```python
from build123d import *

# Parameters (mm, degrees)
F0_W     = 78.4
F0_H     = 24.4
F0_R     = 1
F0_R_2   = 4.1
F1_DEPTH = 1.5
F2_W     = 25
F2_H     = 1.5
F3_DEPTH = 40
F4_R     = 1
F4_R_2   = 4.1
F5_DEPTH = 1.5
F6_R     = 5


with BuildPart() as f1:
    # F0 (on Top) → F1 (new body)
    with BuildSketch(Plane.XY):
        Rectangle(F0_W, F0_H)
        with Locations((-36.2, -7.2)):
            Circle(F0_R, mode=Mode.SUBTRACT)
        with Locations((-4.6, -7.2)):
            Circle(F0_R, mode=Mode.SUBTRACT)
        with Locations((4.6, -7.2)):
            Circle(F0_R, mode=Mode.SUBTRACT)
        with Locations((36.2, -7.2)):
            Circle(F0_R, mode=Mode.SUBTRACT)
        with Locations((-30, 0)):
            Circle(F0_R_2, mode=Mode.SUBTRACT)
        with BuildLine():
            ThreePointArc((-22.5, 4.8), (-21.035534, 8.335534), (-17.5, 9.8))
            Line((-17.5, 9.8), (-7.8, 9.8))
            ThreePointArc((-7.8, 9.8), (-7.092893, 9.507107), (-6.8, 8.8))
            Line((-6.8, 8.8), (-6.8, 5.59017))
            ThreePointArc((-6.8, 5.59017), (-6.712871, 5.181922), (-6.466667, 4.844814))
            ThreePointArc((-6.466667, 4.844814), (-4.3, 0), (-6.466667, -4.844814))
            ThreePointArc((-6.466667, -4.844814), (-6.712871, -5.181922), (-6.8, -5.59017))
            Line((-6.8, -5.59017), (-6.8, -8.8))
            ThreePointArc((-6.8, -8.8), (-7.092893, -9.507107), (-7.8, -9.8))
            Line((-7.8, -9.8), (-17.5, -9.8))
            ThreePointArc((-17.5, -9.8), (-21.035534, -8.335534), (-22.5, -4.8))
            Line((-22.5, -4.8), (-22.5, 4.8))
        make_face(mode=Mode.SUBTRACT)
        with Locations((-36.2, 7.2)):
            Circle(F0_R, mode=Mode.SUBTRACT)
        with Locations((-4.6, 7.2)):
            Circle(F0_R, mode=Mode.SUBTRACT)
        with BuildLine():
            Line((6.8, 5.59017), (6.8, 8.8))
            ThreePointArc((6.8, 8.8), (7.092893, 9.507107), (7.8, 9.8))
            Line((7.8, 9.8), (17.5, 9.8))
            ThreePointArc((17.5, 9.8), (21.035534, 8.335534), (22.5, 4.8))
            Line((22.5, 4.8), (22.5, -4.8))
            ThreePointArc((22.5, -4.8), (21.035534, -8.335534), (17.5, -9.8))
            Line((17.5, -9.8), (7.8, -9.8))
            ThreePointArc((7.8, -9.8), (7.092893, -9.507107), (6.8, -8.8))
            Line((6.8, -8.8), (6.8, -5.59017))
            ThreePointArc((6.8, -5.59017), (6.712871, -5.181922), (6.466667, -4.844814))
            ThreePointArc((6.466667, -4.844814), (4.3, 0), (6.466667, 4.844814))
            ThreePointArc((6.466667, 4.844814), (6.712871, 5.181922), (6.8, 5.59017))
        make_face(mode=Mode.SUBTRACT)
        with Locations((30, 0)):
            Circle(F0_R_2, mode=Mode.SUBTRACT)
        with Locations((4.6, 7.2)):
            Circle(F0_R, mode=Mode.SUBTRACT)
        with Locations((36.2, 7.2)):
            Circle(F0_R, mode=Mode.SUBTRACT)
    extrude(amount=F1_DEPTH)

    # F2 (on Top) → F3 (join)
    with BuildSketch(Plane.XY):
        with Locations((0, 12.95)):
            Rectangle(F2_W, F2_H)
    extrude(amount=F3_DEPTH)

    # F4 (on face) → F5 (cut, through all)
    with BuildSketch(Plane(origin=(0, 13.7, 0), x_dir=(-1, 0, 0), z_dir=(0, 1, 0))):
        with Locations((7.2, 37)):
            Circle(F4_R)
        with Locations((7.2, 5.4)):
            Circle(F4_R)
        with Locations((0, 11.6)):
            Circle(F4_R_2)
        with BuildLine():
            ThreePointArc((9.8, 33.9), (9.507107, 34.607107), (8.8, 34.9))
            Line((8.8, 34.9), (5.499091, 34.9))
            ThreePointArc((5.499091, 34.9), (5.099091, 34.983485), (4.765879, 35.22))
            ThreePointArc((4.765879, 35.22), (0, 37.3), (-4.765879, 35.22))
            ThreePointArc((-4.765879, 35.22), (-5.099091, 34.983485), (-5.499091, 34.9))
            Line((-5.499091, 34.9), (-8.8, 34.9))
            ThreePointArc((-8.8, 34.9), (-9.507107, 34.607107), (-9.8, 33.9))
            Line((-9.8, 33.9), (-9.8, 24.2))
            ThreePointArc((-9.8, 24.2), (-8.335534, 20.664466), (-4.8, 19.2))
            Line((-4.8, 19.2), (4.8, 19.2))
            ThreePointArc((4.8, 19.2), (8.335534, 20.664466), (9.8, 24.2))
            Line((9.8, 24.2), (9.8, 33.9))
        make_face()
        with Locations((-7.2, 37)):
            Circle(F4_R)
        with Locations((-7.2, 5.4)):
            Circle(F4_R)
    extrude(amount=-F5_DEPTH, mode=Mode.SUBTRACT)

    # F6
    f6_edges = [f1.edges().sort_by_distance(p)[0] for p in [
        (-39.2, 12.2, 0.75),
        (-39.2, -12.2, 0.75),
        (39.2, 12.2, 0.75),
        (39.2, -12.2, 0.75),
        (-12.5, 12.95, 40),
        (12.5, 12.95, 40),
    ]]
    fillet(f6_edges, radius=F6_R)


solid = f1.part
```
CAD build for the part. Positions are in the model's coordinates, mm. A direction names the side the tool comes from. Coordinates: 2 decimals unless noted, no trailing zeros. Write each loop counter-clockwise with the first axis right and the second up, starting at its lowest first coordinate (ties: lowest second). Pieces come first, ordered by that corner, then holes.
(1) Cut at A-A, the plane z = 31. List the corners of the cut face in (x, y), and give its area (3 significant figures).
(2) Cut at D-D, the plane z = 5.4. List the corners of the cut face in (x, y).
(3) Cut at C-C, the plane x = 30. List the corners of the cut face in (y, z).
(4) Two-plate mould, pull along Y, no slides. Class faces 4 (the face through (21, 8.37, 0.74)), 5 (the face through (0, 12.2, 16)), 6 (the face through (11, 12.96, 38.57)): +Y half, -Y half, draft (parallel to the pull), parting line (faces both ways), or undercut.
(5) Drill centre lines: probe 1 along Z at (x, y) = (0, 12.8); probe 2 along Y at (x, z) = (-30, 1.1); probe 3 along Z at (x, y) = (7.2, 13.1). Where is each one in solid material? Low to high.
(6) Flat gauge pins, fed straight in: pin 1 (2.5 mm diameter, centred on x = 36.2, y = 7.2, fed in from +Z); pin 2 (10 mm diameter, centred on x = 6.5, z = 21, fed in from -Y). Where does each tip first touch, or does it go through?
(7) Cut at B-B, the plane y = 0. List the corners of the cut face in (x, z), and give its area (3 significant figures).
(8) 3-axis set-ups, long thin cutter, end or side, ignore diameter. For faces 1 (the face through (-1, 0, 1.5)), 2 (the face through (-21, -8.37, 0.74)), 3 (the face through (37.7, -10.77, 0.76)): which of +Z, -Z, +X, -X, +Y, -Y reach the whole face in a straight line?
Geometry says:
1. outline: (-12.5, 12.2) - (-9.8, 12.2) - (-9.8, 13.7) - (-12.5, 13.7) - close; (9.8, 12.2) - (12.5, 12.2) - (12.5, 13.7) - (9.8, 13.7) - close
1. area: 8.10 mm2
2. outline: (-12.5, 12.2) - (-8.2, 12.2) - (-8.2, 13.7) - (-12.5, 13.7) - close; (-6.2, 12.2) - (6.2, 12.2) - (6.2, 13.7) - (-6.2, 13.7) - close; (8.2, 12.2) - (12.5, 12.2) - (12.5, 13.7) - (8.2, 13.7) - close
3. outline: (-12.2, 0) - (-4.1, 0) - (-4.1, 1.5) - (-12.2, 1.5) - close; (4.1, 0) - (12.2, 0) - (12.2, 1.5) - (4.1, 1.5) - close
4. face 4: undercut
4. face 5: -Y half
4. face 6: draft
5. probe 1: z = 0 to 7.5, 15.7 to 19.2, 37.3 to 40
5. probe 2: y = -12.2 to -4.1, 4.1 to 12.2
5. probe 3: z = 0 to 4.4, 6.4 to 19.81, 34.9 to 36, 38 to 40
6. pin 1: stops at z = 1.5
6. pin 2: stops at y = 12.2
7. outline: (-39.2, 0) - (-34.1, 0) - (-34.1, 1.5) - (-39.2, 1.5) - close; (-25.9, 0) - (-22.5, 0) - (-22.5, 1.5) - (-25.9, 1.5) - close; (-4.3, 0) - (4.3, 0) - (4.3, 1.5) - (-4.3, 1.5) - close; (22.5, 0) - (25.9, 0) - (25.9, 1.5) - (22.5, 1.5) - close; (34.1, 0) - (39.2, 0) - (39.2, 1.5) - (34.1, 1.5) - close
7. area: 38.4 mm2
8. face 1: +Z, +X, -X, -Y
8. face 2: +Z, -Z
8. face 3: +Z, -Z, +X, -Y
